Source: three-view drawing plus pictorial views. Frame: mm from the lowest corner of the part. Give positions to 0.01 mm unless a question says otherwise; leave off trailing zeros. Loops run counter-clockwise (first coordinate to the right, second up) from the corner with the lowest first, then second, coordinate; pieces in that order, holes last. Notation, with made-up numbers: (-10, 37) - (8, 37) arc R21 cw to (8, 57) - close; hole circle Ø5 at (-17, -32). An arc over 180 degrees is marked (long way). Answer as a JSON object with one key per item and string values.
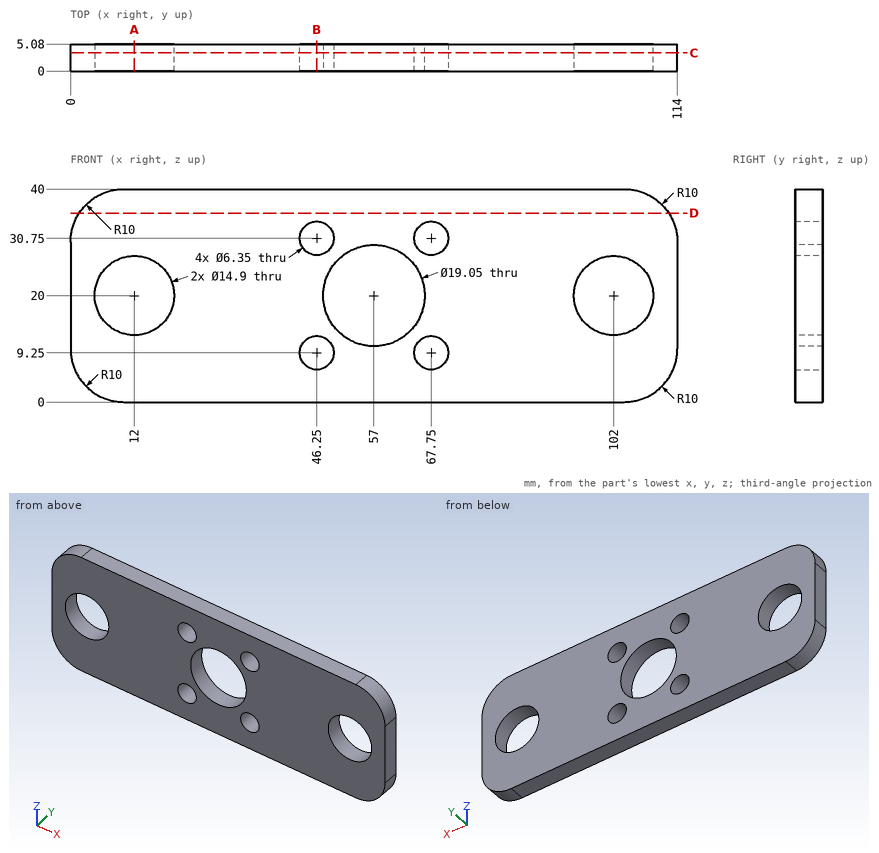
Item 1: Contact query for a flat-ended pin moving along its axis: P1, Ø13.5, axis at x = 102, z = 20, coming from the -Y side. Output: stop coordinate, or through.
Geometry check:
{"P1": "passes through"}
Item 2: Cut plane B-B (x = 46.25). Return loops of the section in (y, z) (3 decimals).
Geometry check:
{"outline": "(0, 0) - (5.08, 0) - (5.08, 6.075) - (0, 6.075) - close; (0, 12.425) - (5.08, 12.425) - (5.08, 27.575) - (0, 27.575) - close; (0, 33.925) - (5.08, 33.925) - (5.08, 40) - (0, 40) - close"}
Item 3: Cut plane C-C (y = 3.4). Return loops of the section in (x, z) (3 decimals), then the cut area to 3 significant figures.
Geometry check:
{"outline": "(0, 10) arc R10 ccw to (10, 0) - (104, 0) arc R10 ccw to (114, 10) - (114, 30) arc R10 ccw to (104, 40) - (10, 40) arc R10 ccw to (0, 30) - close; hole circle Ø14.9 at (12, 20); hole circle Ø6.35 at (46.25, 9.25); hole circle Ø6.35 at (46.25, 30.75); hole circle Ø19.05 at (57, 20); hole circle Ø6.35 at (67.75, 9.25); hole circle Ø6.35 at (67.75, 30.75); hole circle Ø14.9 at (102, 20)", "area": "3,710 mm2"}
Item 4: Cut plane A-A (x = 12). Return loops of the section in (y, z), then the cut area to 3 significant figures.
Geometry check:
{"outline": "(0, 0) - (5.08, 0) - (5.08, 12.55) - (0, 12.55) - close; (0, 27.45) - (5.08, 27.45) - (5.08, 40) - (0, 40) - close", "area": "128 mm2"}
Item 5: Cut plane D-D (z = 35.5). Return loops of the section in (x, y).
Geometry check:
{"outline": "(1.65, 0) - (112.35, 0) - (112.35, 5.08) - (1.65, 5.08) - close"}
Item 6: Material intervals for line 1 (Z direction, x = 46.25, y = 1.8) (3 decimals); line 2 (X direction, y = 3.45, z = 20) (3 decimals); line 3 (X direction, y = 1.3, z = 7.5), sorted ascending. Write a range as [from, to].
Geometry check:
{"line 1": "z = [0, 6.075], [12.425, 27.575], [33.925, 40]", "line 2": "x = [0, 4.55], [19.45, 47.475], [66.525, 94.55], [109.45, 114]", "line 3": "x = [0.32, 43.6], [48.9, 65.1], [70.4, 113.68]"}
